The figure shows three views and two pictorial views of one solid part (mm, origin at its lowest corner). Answer the questions. A direction names the side the tool comes from. Coordinates: 2 decimals unless noted, no trailing zeros. Write each loop counter-clockwise with the first axis right and the second up, starting at its lowest first coordinate (ties: lowest second). Pieces come first, ordered by that corner, then holes. Notation, with made-up numbers: (71.5, 30) - (123.5, 30) arc R17 ccw to (123.5, 40) - close; hole circle Ø5 at (-19, 11.25). An arc over 180 degrees is marked (long way). Use a Markdown table: item, result. Add a question column.
(1) Find the intervals of material crossed by line 1 (Y direction, x = 37, z = 4); line 2 (X direction, y = 46, z = 6); line 3 (X direction, y = 12, z = 5.5), in increasing order. Write a range as from..to.
(2) Given pin 1 Ø6 at (x, y) = (26, 11.5) entering from -Z; pin 2 Ø5 at (y, z) = (32.5, 6) entering from +X; pin 3 Ø3 at (x, z) = (47, 3) entering from +Y; pin 4 Ø5 at (y, z) = (52, 7) entering from +X, each flat-ended and moving along its own axis, determine where each tip first touches the part or whether it passes through.
(3) A tool of negligible diameter and unlimited length cuts with its end or side. For the marked faces 5 and 6, from which of +Z, -Z, +X, -X, +Y, -Y can it reach the whole face along a straight path? Write none if from no direction.
(4) The part is cut by section C-C, the plane z = 7.75. Give the vertices of the cut face in (x, y) (1 decimal).
(5) The part is cut by section D-D, the plane x = 35. Give the vertices of the cut face in (y, z), then the cut area to 3 significant figures.
(6) The part is cut by section B-B, the plane y = 14.5. Give the vertices of the cut face in (x, z).
(7) For a pull along X with two mould halves and no side action, classify the marked faces 1, 2, 3 and 4 as released by +X, released by -X, zero draft, split by the parting line, or undercut.
(8) The part is cut by section A-A, the plane x = 6.5. Give the vertices of the cut face in (y, z).
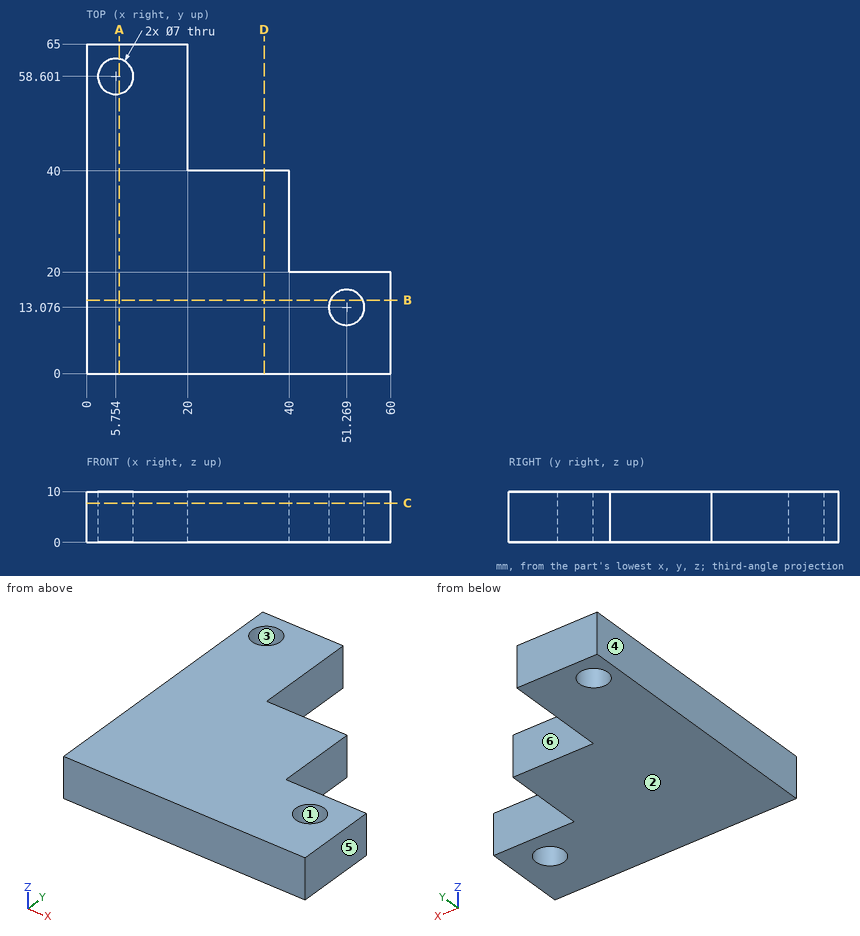
Model answer:
| question | item | result |
|---|---|---|
| 1 | line 1 | 0..40 |
| 1 | line 2 | 0..20 |
| 1 | line 3 | 0..47.94, 54.6..60 |
| 2 | pin 1 | z = 0 |
| 2 | pin 2 | x = 40 |
| 2 | pin 3 | y = 20 |
| 2 | pin 4 | x = 20 |
| 3 | face 5 | +Z, -Z, +X, +Y, -Y |
| 3 | face 6 | +Z, -Z, +X, +Y |
| 4 | outline | (0, 0) - (60, 0) - (60, 20) - (40, 20) - (40, 40) - (20, 40) - (20, 65) - (0, 65) - close; hole circle Ø7 at (5.8, 58.6); hole circle Ø7 at (51.3, 13.1) |
| 5 | outline | (0, 0) - (40, 0) - (40, 10) - (0, 10) - close |
| 5 | area | 400 mm^2 |
| 6 | outline | (0, 0) - (48.07, 0) - (48.07, 10) - (0, 10) - close; (54.47, 0) - (60, 0) - (60, 10) - (54.47, 10) - close |
| 7 | face 1 | undercut |
| 7 | face 2 | zero draft |
| 7 | face 3 | undercut |
| 7 | face 4 | released by -X |
| 8 | outline | (0, 0) - (55.18, 0) - (55.18, 10) - (0, 10) - close; (62.02, 0) - (65, 0) - (65, 10) - (62.02, 10) - close |
